from build123d import *

# Parameters (mm, degrees)
SKETCH1_R           = 10.5
BOSS_EXTRUDE1_DEPTH = 40.5
SKETCH2_W           = 41.275373403
SKETCH2_H           = 50.56233242
CUT_EXTRUDE1_DEPTH  = 40.5
SHELL3_T            = -1


with BuildPart() as part:
    # Sketch1 → Boss-Extrude1 (new body)
    with BuildSketch(Plane(origin=(0, 0, 0), x_dir=(1, 0, 0), z_dir=(0, 1, 0))):
        with Locations(Location((0, 0, 0), (0, 0, 270))):
            Circle(SKETCH1_R)
    extrude(amount=BOSS_EXTRUDE1_DEPTH)

    # Sketch2 → Cut-Extrude1 (cut)
    with BuildSketch(Plane(origin=(0, 0, 0), x_dir=(0, 0, -1), z_dir=(1, 0, 0))):
        with Locations((2.800828909, 23.566771077)):
            Rectangle(SKETCH2_W, SKETCH2_H)
    extrude(amount=-CUT_EXTRUDE1_DEPTH, mode=Mode.SUBTRACT)

    # Shell3
    shell3_openings = [part.faces().sort_by_distance(p)[0] for p in [
        (4.456338407, 40.5, 0),
        (0, 20.25, 0),
    ]]
    offset(amount=SHELL3_T, openings=shell3_openings)


solid = part.part
Design review of the part built by this model. Coordinates are the model's own, in mm. Give positions to 0.01 mm unless a question says otherwise; leave off trailing zeros. Order: outer loops, then holes, each group sorted by start corner. A loop starts at its lowest first (then second) coordinate and runs counter-clockwise, first axis right, second up.
1. Add section A-A, the plane x = 6.75. State the section outline as (y, z) points, then the cut area to 3 significant figures.
Solution:
outline: (0, -8.04) - (40.5, -8.04) - (40.5, -6.68) - (1, -6.68) - (1, 6.68) - (40.5, 6.68) - (40.5, 8.04) - (0, 8.04) - close
area: 123 mm2
2. For pin 1 Ø1 at (x, z) = (3, 4.5) entering from -Y; pin 2 Ø1.5 at (y, z) = (6.5, 4.5) entering from +X; pin 3 Ø2 at (y, z) = (32.5, 2.5) entering from +X; pin 4 Ø5 at (y, z) = (14, -7.5) entering from +X, all flat-tipped, find the tip position at first contact; note any pin that passes through.
Solution:
pin 1: stops at y = 0
pin 2: stops at x = 9.81
pin 3: stops at x = 10.39
pin 4: stops at x = 9.23
3. Add section D-D, the plane x = 2.25. State the section outline as (y, z) points.
Solution:
outline: (0, -10.26) - (40.5, -10.26) - (40.5, -9.23) - (1, -9.23) - (1, 9.23) - (40.5, 9.23) - (40.5, 10.26) - (0, 10.26) - close
4. Mouldability with a two-part tool opening along Z and no side actions: class faces 1 (the flat face through (4, 0, 0)), 2 (the cylindrical face through (9.498, 20.474, 0.209)), 3 (the cylindrical face through (10.5, 20, 0.2)), 4 (the flat face through (4, 1, 0)) as +Z half, -Z half, draft (parallel to the pull), parting line (faces both ways), or undercut.
Solution:
face 1: draft
face 2: undercut
face 3: parting line
face 4: undercut
5. Add section B-B, the plane z = 0. State the section outline as (x, y) points, then the cut area to 3 significant figures.
Solution:
outline: (0, 0) - (10.5, 0) - (10.5, 40.5) - (9.5, 40.5) - (9.5, 1) - (0, 1) - close
area: 50.0 mm2
6. Add section C-C, the plane y = 18. State the section outline as (x, z) points, then the cut area to 3 significant figures.
Solution:
outline: (0, -10.5) arc R10.5 ccw to (0, 10.5) - (0, 9.5) arc R9.5 cw to (0, -9.5) - close
area: 31.4 mm2
7. To check wall thickness, follow L1, parallel to Y at x = 4.5, z = 1.25; L2, parallel to Z at x = 3.25, y = 31; L3, parallel to Z at x = 5.5, y = 37. State the ranges of each line that lie inside material, in increasing order.
Solution:
L1: y = 0 to 1
L2: z = -9.98 to -8.93, 8.93 to 9.98
L3: z = -8.94 to -7.75, 7.75 to 8.94
